Input: part model. Units: mm. Frame: model coordinates. A direction names the side the tool comes from. Give positions to 0.01 mm unless a question says otherwise; leave off trailing zeros. Write each loop counter-clockwise with the first axis right and the second up, starting at its lowest first coordinate (ties: lowest second). Pieces come first, ordered by that corner, then holes. Notation, with made-up numbers: (-35.5, -1) - (-9.5, -1) arc R15 ccw to (-9.5, 28) - close; hole circle Ø4 at (76, -8.75). An arc over 180 degrees is marked (long way). Answer as CSV lines item,"result".
```python
from build123d import *

# Parameters (mm, degrees)
SKETCH_1_W       = 320
SKETCH_1_H       = 110
EXTRUDE_1_DEPTH  = 55
SHELL_1_T        = -5
RIB_1_REACH      = 179.904
SKETCH_2_WALLS_W = 5
SKETCH_2_WALLS_H = 457.808937494


with BuildPart() as part:
    # 草图1 → 凸台-拉伸1 (new body)
    with BuildSketch(Plane(origin=(0, 0, 0), x_dir=(1, 0, 0), z_dir=(0, 1, 0))):
        Rectangle(SKETCH_1_W, SKETCH_1_H)
    extrude(amount=EXTRUDE_1_DEPTH)

    # 抽壳1
    shell_1_openings = [part.faces().sort_by_distance(p)[0] for p in [
        (0, 55, 0),
    ]]
    offset(amount=SHELL_1_T, openings=shell_1_openings, kind=Kind.INTERSECTION)

    # 草图2 walls → 筋1 (add, up to next)
    with BuildSketch(Plane(origin=(0, 55, 0), x_dir=(1, 0, 0), z_dir=(0, 1, 0)), mode=Mode.PRIVATE) as rib_1_sk1:
        with Locations((52.5, 0)):
            Rectangle(SKETCH_2_WALLS_W, SKETCH_2_WALLS_H)
    rib_1_tool1 = extrude(rib_1_sk1.sketch, amount=-RIB_1_REACH, mode=Mode.PRIVATE) - part.part
    # 草图2 walls → 筋1 (add, up to next)
    with BuildSketch(Plane(origin=(0, 55, 0), x_dir=(1, 0, 0), z_dir=(0, 1, 0)), mode=Mode.PRIVATE) as rib_1_sk2:
        with Locations((-52.5, 0)):
            Rectangle(SKETCH_2_WALLS_W, SKETCH_2_WALLS_H)
    rib_1_tool2 = extrude(rib_1_sk2.sketch, amount=-RIB_1_REACH, mode=Mode.PRIVATE) - part.part
    add(rib_1_tool1.solids().sort_by_distance((52.5, 55, 0))[0])
    add(rib_1_tool2.solids().sort_by_distance((-52.5, 55, 0))[0])


solid = part.part
```
Item 1: Reachability of faces 1 (the face through (-55, 30, 1)), 2 (the face through (-160, 27, 1)) from +Z, -Z, +X, -X, +Y, -Y: full face, straight path, thin tool, end or side. Return the list, or none.
The answers:
face 1,"+Y"
face 2,"+Z, -Z, -X, +Y, -Y"
Item 2: Cut plane B-B on x = 127. Return the cut outline in (y, z), plus the area to 3 significant figures.
The answers:
outline,"(0, -55) - (55, -55) - (55, -50) - (5, -50) - (5, 50) - (55, 50) - (55, 55) - (0, 55) - close"
area,"1,050 mm²"
Item 3: Ray query, line 1 (X direction, y = 35.5, z = -7.5); line 2 (Z direction, x = 1.5, y = 44); line 3 (Y direction, x = -140.5, z = 26). Return the intervals inside material, ascending. Write a range as from..to.
The answers:
line 1,"-160..-155, -55..-50, 50..55, 155..160"
line 2,"-55..-50, 50..55"
line 3,"0..5"
Item 4: Cut plane A-A on y = 36. Return the cut outline in (x, z).
The answers:
outline,"(-160, -55) - (160, -55) - (160, 55) - (-160, 55) - close; hole (-155, -50) - (-55, -50) - (-55, 50) - (-155, 50) - close; hole (-50, -50) - (50, -50) - (50, 50) - (-50, 50) - close; hole (55, -50) - (155, -50) - (155, 50) - (55, 50) - close"
Item 5: Contact query for a flat-ended pin moving along its axis: pin 1 (4 mm diameter, centred on x = 18, z = 17, fed in from +Y). Output: stop coordinate, or through.
The answers:
pin 1,"y = 5"
Item 6: Cut plane C-C on z = 24. Return the cut outline in (x, y), plus the area to 3 significant figures.
The answers:
outline,"(-160, 0) - (160, 0) - (160, 55) - (155, 55) - (155, 5) - (55, 5) - (55, 55) - (50, 55) - (50, 5) - (-50, 5) - (-50, 55) - (-55, 55) - (-55, 5) - (-155, 5) - (-155, 55) - (-160, 55) - close"
area,"2,600 mm²"
Item 7: Mould query, pull axis Z, two halves, no side actions, for faces 3 (the face through (160, 27, 1)), 4 (the face through (155, 30, 1)), 5 (the face through (104, 30, 50)), 6 (the face through (-2, 27, 55)). Classes: +Z half, -Z half, draft (parallel to the pull), parting line (faces both ways), or undercut.
The answers:
face 3,"draft"
face 4,"undercut"
face 5,"undercut"
face 6,"+Z half"
